Autodesk Fusion 360 part; units mm, degrees
sketch "Sketch1" plane through (0, 0, 0) normal (0, 1, 0) x (1, 0, 0)
  line L0 (-12.1, -17.5) -> (-13.8, 0)
  line L1 (-12.1, -17.5) -> (-11.5171, -23.5)
  line L2 (-13.8, 0) -> (0, 0)
  line L3 (0, 0) -> (0, -23.5) construction
  line L4 (-12.1, -17.5) -> (0, -17.5) construction
  line L5 (-11.5171, -23.5) -> (0, -23.5)
  line L6 (0, 0) -> (0, -23.5) construction
  line L7 (13.8, 0) -> (0, 0)
  line L8 (12.1, -17.5) -> (13.8, 0)
  line L9 (11.5171, -23.5) -> (0, -23.5)
  line L10 (12.1, -17.5) -> (11.5171, -23.5)
  line L11 (0, -29.5) -> (33.5, 4) construction
  line L12 (33.5, 4) -> (33.5, 7.6922)
  line L13 (0, -29.5) -> (14.1, -29.5)
  line L14 (14.1, -29.5) -> (14.1, -15.4)
  line L15 (0, -29.5) -> (-14.1, -29.5)
  line L16 (-14.1, -29.5) -> (-14.1, -15.4)
  line L17 (14.1, -15.4) -> (-14.1, -15.4)
  line L18 (33.5, 4) -> (28.0093, 4)
  line L19 (28.0093, 4) -> (0, 4)
  line L20 (0, 4) -> (0, -29.5)
  line L21 (3, -29.5) -> (33.5, 4)
  line L22 (13.8, 0) -> (16.1094, 4)
  line L23 (-13.8, 0) -> (-16.1094, 4)
  line L24 (-28.0093, 4) -> (0, 4)
  dimension "d1" = 17.5
  dimension "d4" = 6
  dimension "d7" = 27.6
  dimension "d8" = 24.2
  dimension "d13" = 135
  dimension "d14" = 2
  dimension "d15" = 6
  dimension "d16" = 4
  dimension "d22" = 3
  dimension "d26" = 60
extrude "Extrude1" add sketch "Sketch1" along normal mid plane 6.1 contours L0 L1 L5 L17 L20 | L0 L2 L17 L20 | L2 L20 L23 L24 | L7 L8 L17 L20 | L8 L9 L10 L17 L20 L21 | L7 L19 L20 L22 | L9 L10 L21 makes body 1
fillet "Fillet1" radius 0.4 2 edges at (11.5171, 0, 23.5) (-11.5171, 0, 23.5) on bodies 1
revolve "Revolve1" add sketch "Sketch1" angle 360 about axis through (0, 0, -4) along (0, 0, 1) separate body contours L7 L8 L17 L20 | L8 L9 L10 L17 L20 L21 | L9 L13 L20 L21 | L7 L19 L20 L22 | L8 L10 L14 L17 L21 | L8 L14 L17 L18 L19 L21 L22 makes body 2
sketch "Sketch3" plane through (0, 0, -4) normal (0, 0, -1) x (1, 0, 0)
  circle A0 centre (0, 0) radius 33.5
  line L0 (-16.1094, 3.05) -> (-16.1094, -3.05) construction
  line L1 (-16.1094, -3.05) -> (16.1094, -3.05) construction
  line L2 (16.1094, -3.05) -> (16.1094, 3.05) construction
  line L3 (16.1094, 3.05) -> (-16.1094, 3.05) construction
  line L4 (18.1094, 5.05) -> (-18.1094, 5.05)
  line L5 (-18.1094, 5.05) -> (-18.1094, -5.05)
  line L6 (-18.1094, -5.05) -> (18.1094, -5.05)
  line L7 (18.1094, -5.05) -> (18.1094, 5.05)
  dimension "d27" = 2
extrude "Extrude3" add sketch "Sketch3" against normal blind 40 contours L4 L5 L6 L7 bodies 2
combine "Combine1" operation cut target body 2 tool bodies 1
chamfer "Chamfer1" distance 2 angle 45 2 edges at (18.1094, 0, 36) (-18.1094, 0, 36) on bodies 2
sketch "Sketch4" plane through (0, 0, 0) normal (0, 1, 0) x (1, 0, 0)
  line L0 (18.1094, -12.9044) -> (33.5, 4)
  line L1 (-33.5, 4) -> (-18.1094, -12.9044)
  line L2 (33.5, 4) -> (27.5, 4)
  line L3 (27.5, 4) -> (23.8582, 0)
  line L4 (23.8582, 0) -> (0, 0)
  line L5 (0, 0) -> (0, 4)
  line L6 (0, 4) -> (27.5, 4)
  point P0 (-33.5, 4)
  point P1 (33.5, 4)
  dimension "d29" = 6
revolve "Revolve2" cut sketch "Sketch4" angle 360 about axis through (0, 0, 1.75) along (0, 0, 1) bodies 2
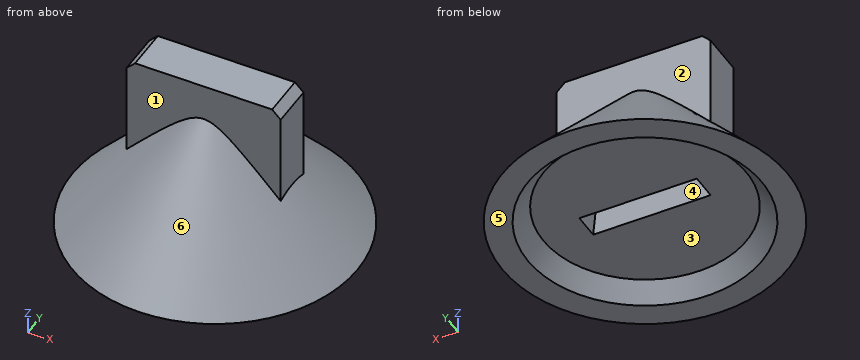
Build history of the part. All positions in model axes, mm. Face numbers are marked on the shaded views. A direction names the side the tool comes from. Give positions to 0.01 mm unless a question says otherwise; leave off trailing zeros. Loops run counter-clockwise (first coordinate to the right, second up) from the corner with the lowest first, then second, coordinate; pieces in that order, holes last. Notation, with made-up numbers: (-27, 25.5) -> (-13, 25.5) arc R28 cw to (-13, 52.5) -> close; hole circle Ø10 at (24, 52.25). An arc over 180 degrees is marked (long way). One line per question, with ' | ' between items.
Q1. Cut at D-D, the plane z = 29.5. Write the cut outline in (x, y), plus the area to 3 significant figures.
Filled sheet:
outline: (-18.11, -5.05) -> (18.11, -5.05) -> (18.11, 5.05) -> (-18.11, 5.05) -> close | area: 366 mm²
Q2. Cut at C-C, the plane x = 0. Write the cut outline in (y, z), plus the area to 3 significant figures.
Filled sheet:
outline: (-33.5, -4) -> (-27.5, -4) -> (-23.86, 0) -> (-3.05, 0) -> (-3.05, 23.5) -> (3.05, 23.5) -> (3.05, 0) -> (23.86, 0) -> (27.5, -4) -> (33.5, -4) -> (5.05, 27.25) -> (5.05, 36) -> (-5.05, 36) -> (-5.05, 27.25) -> close | area: 944 mm²
Q3. Cut at A-A, the plane y = 0. Write the cut outline in (x, z).
Filled sheet:
outline: (-33.5, -4) -> (-27.5, -4) -> (-23.86, 0) -> (-13.8, 0) -> (-12.1, 17.5) -> (-11.55, 23.14) arc R0.4 cw to (-11.15, 23.5) -> (11.15, 23.5) arc R0.4 cw to (11.55, 23.14) -> (12.1, 17.5) -> (13.8, 0) -> (23.86, 0) -> (27.5, -4) -> (33.5, -4) -> (18.11, 12.9) -> (18.11, 34) -> (16.11, 36) -> (-16.11, 36) -> (-18.11, 34) -> (-18.11, 12.9) -> close
Q4. Drop flat-ended pins along their axis: pin 1 (2 mm diameter, centred on x = 13, z = 8.5, fed in from -Y); pin 2 (24 mm diameter, centred on x = 7, y = 1, fed in from -Z); pin 3 (5 mm diameter, centred on y = -5, z = 17.5, fed in from -X). Give the stop position or say it passes through.
Filled sheet:
pin 1: stops at y = -19.2 | pin 2: stops at z = 0 | pin 3: stops at x = -18.11
Q5. Pull direction Y, two halves, no side cores. Call the marked faces 4, 5 and 6: pulls with the +Y half, pulls with the -Y half, needs draft (parallel to the pull), parting line crosses it, or undercut.
Filled sheet:
face 4: undercut | face 5: needs draft | face 6: parting line crosses it
Q6. Drill centre lines: line 1 along Y through (x, z) = (10.5, 21); line 2 along Y through (x, z) = (-19.5, 5); line 3 along Y through (x, z) = (-6, 10). Where is each one in solid material? Low to high. Write a range as [from, to].
Filled sheet:
line 1: y = [-5.05, -3.05], [3.05, 5.05] | line 2: y = [-16.13, 16.13] | line 3: y = [-19.87, -3.05], [3.05, 19.87]
Q7. Cut at B-B, the plane z = 5.5. Write the cut outline in (x, y).
Filled sheet:
outline: circle Ø49.7 at (0, 0); hole (-13.27, -3.05) -> (13.27, -3.05) -> (13.27, 3.05) -> (-13.27, 3.05) -> close
Q8. Tool access for the marked faces 1, 2 and 3: list every direction of +Z, -Z, +X, -X, +Y, -Y with a clear straight run to the whole face (end or side of a thin tool).
Filled sheet:
face 1: +Z, -Y | face 2: +Z, +Y | face 3: -Z
